For this review, take the finished solid that the model builds, in its own axes (mm). A direction names the side the tool comes from. Coordinates: 2 decimals unless noted, no trailing zeros. Write each loop counter-clockwise with the first axis right and the second up, starting at its lowest first coordinate (ties: lowest second). Pieces come first, ordered by that corner, then holes. Notation, with made-up numbers: (47.5, 12.5) -> (68.5, 12.5) arc R24 cw to (68.5, 42.5) -> close; hole circle Ø1 at (46.5, 26). An arc over 180 degrees is marked (long way). Put each result on its own line as item: value. Start each with the question number.
Item 1: Consider section A-A on x = -31.5. Give the boundary of the cut face in (y, z) (1 decimal), and give its area (3 significant figures).
Item 2: Consider section B-B on z = -3.5. Give the boundary of the cut face in (x, y) (3 decimals), and give its area (3 significant figures).
Item 3: To check wall thickness, follow L1, parallel to Z at x = 13, y = 73; L2, parallel to Z at x = 58.5, y = 20.5 (3 decimals); L3, parallel to Y at x = 14, z = 5 (3 decimals). State the ranges of each line that lie inside material, in increasing order.
Item 4: Consider section C-C on x = -55.5. Give the boundary of the cut face in (y, z) (3 decimals).
Item 5: For faces 1 (the flat face through (38, 1, 9.525)), 2 (the flat face through (-1, 96, 47.964)), 3 (the cylindrical face through (-18.961, 29.851, 58.296)), list the 3-axis set-ups (+Z, -Z, +X, -X, +Y, -Y) from which the entire face can be reached by the end or side of a thin tool; tool diameter is ignored.
Item 6: Insertion check: P1, Ø12, axis at x = -40.5, y = 108, coming from the -Z side; P2, Ø13.5, axis at y = 35, z = 48, coming from the -X side; P3, Ø8, axis at y = 38, z = 32.5, coming from the +X side. Each pin has a flat end and moves straight along its axis. Give the tip position at first contact, or say it passes through.
```python
from build123d import *

# Parameters (mm, degrees)
F1_DEPTH = 63.5
F2_DEPTH = 25.4
F3_DEPTH = 12.7


with BuildPart() as f1:
    # F0 (on Right) → F1 (new body, symmetric)
    with BuildSketch(Plane.YZ):
        Polygon((22.225, 9.525), (-41.275, 9.525), (-41.275, -9.525), (41.275, -9.525), (41.275, 9.525), align=None)
    extrude(amount=F1_DEPTH, both=True)

    # F0 (on Right) → F2 (join, symmetric)
    with BuildSketch(Plane.YZ):
        with BuildLine():
            Line((22.225, 36.5125), (22.225, 9.525))
            Line((22.225, 9.525), (41.275, 9.525))
            Line((41.275, 9.525), (41.275, 36.5125))
            ThreePointArc((41.275, 36.5125), (45.92468, 47.73782), (57.15, 52.3875))
            Line((57.15, 52.3875), (92.761105, 52.3875))
            Line((92.761105, 52.3875), (92.761105, 71.4375))
            Line((92.761105, 71.4375), (57.15, 71.4375))
            ThreePointArc((57.15, 71.4375), (32.454296, 61.208204), (22.225, 36.5125))
        make_face()
    extrude(amount=F2_DEPTH, both=True)

    # F0 (on Right) → F3 (join, symmetric)
    with BuildSketch(Plane.YZ):
        with BuildLine():
            add(Edge.make_bspline(
                [(-41.275, 9.525), (-37.458211, 92.56649), (0, 82.461342), (92.761105, 76.538539)],
                knots=[0, 0, 0, 0, 149.854902, 149.854902, 149.854902, 149.854902], degree=3))
            Line((-41.275, 9.525), (22.225, 9.525))
            Line((22.225, 9.525), (22.225, 36.5125))
            ThreePointArc((22.225, 36.5125), (32.454296, 61.208204), (57.15, 71.4375))
            Line((57.15, 71.4375), (92.761105, 71.4375))
            Line((92.761105, 71.4375), (92.761105, 76.538539))
        make_face()
    extrude(amount=F3_DEPTH, both=True)

    # F0 (on Right) → F4 (revolve)
    with BuildSketch(Plane.YZ):
        Polygon((143.561105, 76.538539), (92.761105, 76.538539), (92.761105, 71.4375), (92.761105, 52.3875), (92.761105, 47.963539), (143.561105, 47.963539), align=None)
    revolve(axis=Axis((0, 92.761105, 62.251039), (0, 0, 1)))


solid = f1.part
```
Return value:
1. outline: (-41.3, -9.5) -> (41.3, -9.5) -> (41.3, 9.5) -> (-41.3, 9.5) -> close; (52.9, 48) -> (132.6, 48) -> (132.6, 76.5) -> (52.9, 76.5) -> close
1. area: 3,850 mm^2
2. outline: (-63.5, -41.275) -> (63.5, -41.275) -> (63.5, 41.275) -> (-63.5, 41.275) -> close
2. area: 10,500 mm^2
3. L1: 47.96 to 76.54
3. L2: -9.525 to 9.525
3. L3: -41.275 to 41.275
4. outline: (-41.275, -9.525) -> (41.275, -9.525) -> (41.275, 9.525) -> (-41.275, 9.525) -> close
5. face 1: +Z, +X, -Y
5. face 2: -Z, +X, -X, +Y
5. face 3: +Z, -X, -Y
6. P1: z = 47.96
6. P2: x = -25.4
6. P3: x = 25.4
